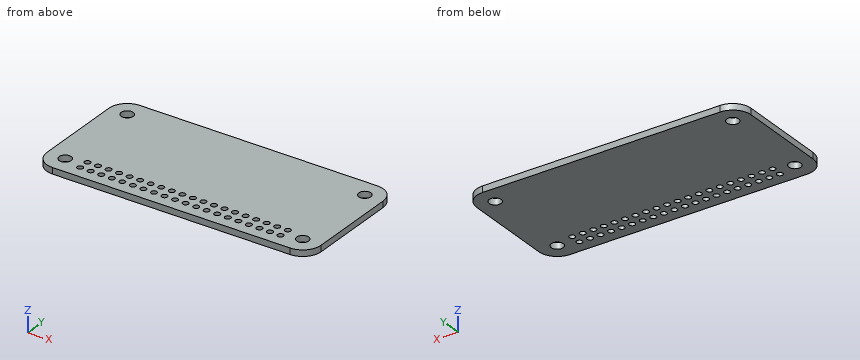
from build123d import *

# Parameters (mm, degrees)
CROQUIS1_R              = 1.45
CROQUIS1_R_2            = 0.7
SALIENTE_EXTRUIR1_DEPTH = 1.5


with BuildPart() as part:
    # Croquis1 → Saliente-Extruir1 (new body)
    with BuildSketch(Plane.XY):
        with BuildLine():
            Line((28.62, -15.24), (-28.62, -15.24))
            ThreePointArc((-28.62, -15.24), (-31.731269837, -13.951269837), (-33.02, -10.84))
            Line((-33.02, -10.84), (-33.02, 10.84))
            ThreePointArc((-33.02, 10.84), (-31.731269837, 13.951269837), (-28.62, 15.24))
            Line((-28.62, 15.24), (28.62, 15.24))
            ThreePointArc((28.62, 15.24), (31.731269837, 13.951269837), (33.02, 10.84))
            Line((33.02, 10.84), (33.02, -10.84))
            ThreePointArc((33.02, -10.84), (31.731269837, -13.951269837), (28.62, -15.24))
        make_face()
        with Locations((-28.62, 10.84)):
            Circle(CROQUIS1_R, mode=Mode.SUBTRACT)
        with Locations(Location((28.62, 10.84, 0), (0, 0, 180))):
            Circle(CROQUIS1_R, mode=Mode.SUBTRACT)
        with Locations((28.62, -10.84)):
            Circle(CROQUIS1_R, mode=Mode.SUBTRACT)
        with Locations(Location((-28.62, -10.84, 0), (0, 0, 180))):
            Circle(CROQUIS1_R, mode=Mode.SUBTRACT)
        with Locations((-24.13, -9.57)):
            Circle(CROQUIS1_R_2, mode=Mode.SUBTRACT)
        with Locations((-24.13, -12.11)):
            Circle(CROQUIS1_R_2, mode=Mode.SUBTRACT)
        with Locations((-21.59, -9.57)):
            Circle(CROQUIS1_R_2, mode=Mode.SUBTRACT)
        with Locations((-21.59, -12.11)):
            Circle(CROQUIS1_R_2, mode=Mode.SUBTRACT)
        with Locations((-19.05, -9.57)):
            Circle(CROQUIS1_R_2, mode=Mode.SUBTRACT)
        with Locations((-19.05, -12.11)):
            Circle(CROQUIS1_R_2, mode=Mode.SUBTRACT)
        with Locations((-16.51, -9.57)):
            Circle(CROQUIS1_R_2, mode=Mode.SUBTRACT)
        with Locations((-16.51, -12.11)):
            Circle(CROQUIS1_R_2, mode=Mode.SUBTRACT)
        with Locations((-13.97, -9.57)):
            Circle(CROQUIS1_R_2, mode=Mode.SUBTRACT)
        with Locations((-13.97, -12.11)):
            Circle(CROQUIS1_R_2, mode=Mode.SUBTRACT)
        with Locations((-11.43, -9.57)):
            Circle(CROQUIS1_R_2, mode=Mode.SUBTRACT)
        with Locations((-11.43, -12.11)):
            Circle(CROQUIS1_R_2, mode=Mode.SUBTRACT)
        with Locations((-8.89, -9.57)):
            Circle(CROQUIS1_R_2, mode=Mode.SUBTRACT)
        with Locations((-8.89, -12.11)):
            Circle(CROQUIS1_R_2, mode=Mode.SUBTRACT)
        with Locations((-6.35, -9.57)):
            Circle(CROQUIS1_R_2, mode=Mode.SUBTRACT)
        with Locations((-6.35, -12.11)):
            Circle(CROQUIS1_R_2, mode=Mode.SUBTRACT)
        with Locations((-3.81, -9.57)):
            Circle(CROQUIS1_R_2, mode=Mode.SUBTRACT)
        with Locations((-3.81, -12.11)):
            Circle(CROQUIS1_R_2, mode=Mode.SUBTRACT)
        with Locations((-1.27, -9.57)):
            Circle(CROQUIS1_R_2, mode=Mode.SUBTRACT)
        with Locations((-1.27, -12.11)):
            Circle(CROQUIS1_R_2, mode=Mode.SUBTRACT)
        with Locations((1.27, -9.57)):
            Circle(CROQUIS1_R_2, mode=Mode.SUBTRACT)
        with Locations((1.27, -12.11)):
            Circle(CROQUIS1_R_2, mode=Mode.SUBTRACT)
        with Locations((3.81, -9.57)):
            Circle(CROQUIS1_R_2, mode=Mode.SUBTRACT)
        with Locations((3.81, -12.11)):
            Circle(CROQUIS1_R_2, mode=Mode.SUBTRACT)
        with Locations((6.35, -9.57)):
            Circle(CROQUIS1_R_2, mode=Mode.SUBTRACT)
        with Locations((6.35, -12.11)):
            Circle(CROQUIS1_R_2, mode=Mode.SUBTRACT)
        with Locations((8.89, -9.57)):
            Circle(CROQUIS1_R_2, mode=Mode.SUBTRACT)
        with Locations((8.89, -12.11)):
            Circle(CROQUIS1_R_2, mode=Mode.SUBTRACT)
        with Locations((11.43, -9.57)):
            Circle(CROQUIS1_R_2, mode=Mode.SUBTRACT)
        with Locations((11.43, -12.11)):
            Circle(CROQUIS1_R_2, mode=Mode.SUBTRACT)
        with Locations((13.97, -9.57)):
            Circle(CROQUIS1_R_2, mode=Mode.SUBTRACT)
        with Locations((13.97, -12.11)):
            Circle(CROQUIS1_R_2, mode=Mode.SUBTRACT)
        with Locations((16.51, -9.57)):
            Circle(CROQUIS1_R_2, mode=Mode.SUBTRACT)
        with Locations((16.51, -12.11)):
            Circle(CROQUIS1_R_2, mode=Mode.SUBTRACT)
        with Locations((19.05, -9.57)):
            Circle(CROQUIS1_R_2, mode=Mode.SUBTRACT)
        with Locations((19.05, -12.11)):
            Circle(CROQUIS1_R_2, mode=Mode.SUBTRACT)
        with Locations((21.59, -9.57)):
            Circle(CROQUIS1_R_2, mode=Mode.SUBTRACT)
        with Locations((21.59, -12.11)):
            Circle(CROQUIS1_R_2, mode=Mode.SUBTRACT)
        with Locations((24.13, -9.57)):
            Circle(CROQUIS1_R_2, mode=Mode.SUBTRACT)
        with Locations((24.13, -12.11)):
            Circle(CROQUIS1_R_2, mode=Mode.SUBTRACT)
    extrude(amount=SALIENTE_EXTRUIR1_DEPTH)


solid = part.part
Input: part model. Units: mm. Frame: model coordinates. Round coordinates to 2 decimals unless told otherwise and drop trailing zeros. Order: outer loops, then holes, each group sorted by start corner. A loop starts at its lowest first (then second) coordinate and runs counter-clockwise, first axis right, second up.
1. Cut plane B-B, the plane z = 0.3. State how many separate pieces and enclosed holes the cut face has, then the cut area to 3 significant figures.
The answers:
separate pieces: 1
enclosed holes: 44
area: 1,910 mm2
2. Cut plane A-A, the plane x = -1.27. Output: boundary loops of the cut face in (y, z), then the cut area to 3 significant figures.
The answers:
outline: (-15.24, 0) - (-12.81, 0) - (-12.81, 1.5) - (-15.24, 1.5) - close; (-11.41, 0) - (-10.27, 0) - (-10.27, 1.5) - (-11.41, 1.5) - close; (-8.87, 0) - (15.24, 0) - (15.24, 1.5) - (-8.87, 1.5) - close
area: 41.5 mm2
3. Material intervals for line 1 (Y direction, x = 8.89, z = 0.75); line 2 (X direction, y = -11, z = 0.55); line 3 (Y direction, x = 19.5, z = 0.7), sorted ascending.
The answers:
line 1: y = -15.24 to -12.81, -11.41 to -10.27, -8.87 to 15.24
line 2: x = -33.02 to -30.06, -27.18 to 27.18, 30.06 to 33.02
line 3: y = -15.24 to -12.65, -11.57 to -10.11, -9.03 to 15.24
4. Pin query (flat end, axial travel): P1, Ø4, axis at x = -28.62, y = 10.84, coming from the +Z side. Return the tip coordinate at first contact, or that it passes through.
The answers:
P1: stops at z = 1.5
